Part print with two shaded views. Sizes in mm from the minimum x, y, z corner. A direction names the side the tool comes from. Coordinates: 2 decimals unless noted, no trailing zeros. Write each loop counter-clockwise with the first axis right and the second up, starting at its lowest first coordinate (ties: lowest second). Pieces come first, ordered by that corner, then holes. Notation, with made-up numbers: (10.5, 29.5) - (33.5, 29.5) arc R9 ccw to (33.5, 41.5) - close; hole circle Ø7 at (51.5, 13.5). An arc over 180 degrees is marked (long way). One line per question, with ' | ' between items. Start each with the question number.
1. Probe line 1 (X direction, y = 2.9, z = 3); line 2 (Z direction, x = 69, y = 2.2); line 3 (X direction, y = 2.25, z = 2.5). List the from-to ranges inside material, lowest first.
2. Which spindle directions (+Z, -Z, +X, -X, +Y, -Y) get a long thin tool onto all of the face, cutting with end or side? Do the marked faces 1, 2 and 3. Say none if no direction does.
3. Band-saw the part on C-C, the plane y = 20.75. Write the cut outline in (x, z), then the cut area to 3 significant figures.
4. Flat gauge pins, fed straight in: P1, Ø1.8, axis at x = 4, z = 3, coming from the +Y side; P2, Ø6.5, axis at y = 17, z = 2.5, coming from the -X side; P3, Ø3, axis at x = 3.5, y = 18, coming from the -Z side. Where does each tip first touch, or does it go through?
5. Band-saw the part on A-A, the plane x = 3. Write the cut outline in (y, z), then the cut area to 3 significant figures.
6. Band-saw the part on B-B, the plane z = 47. Write the cut outline in (x, y).
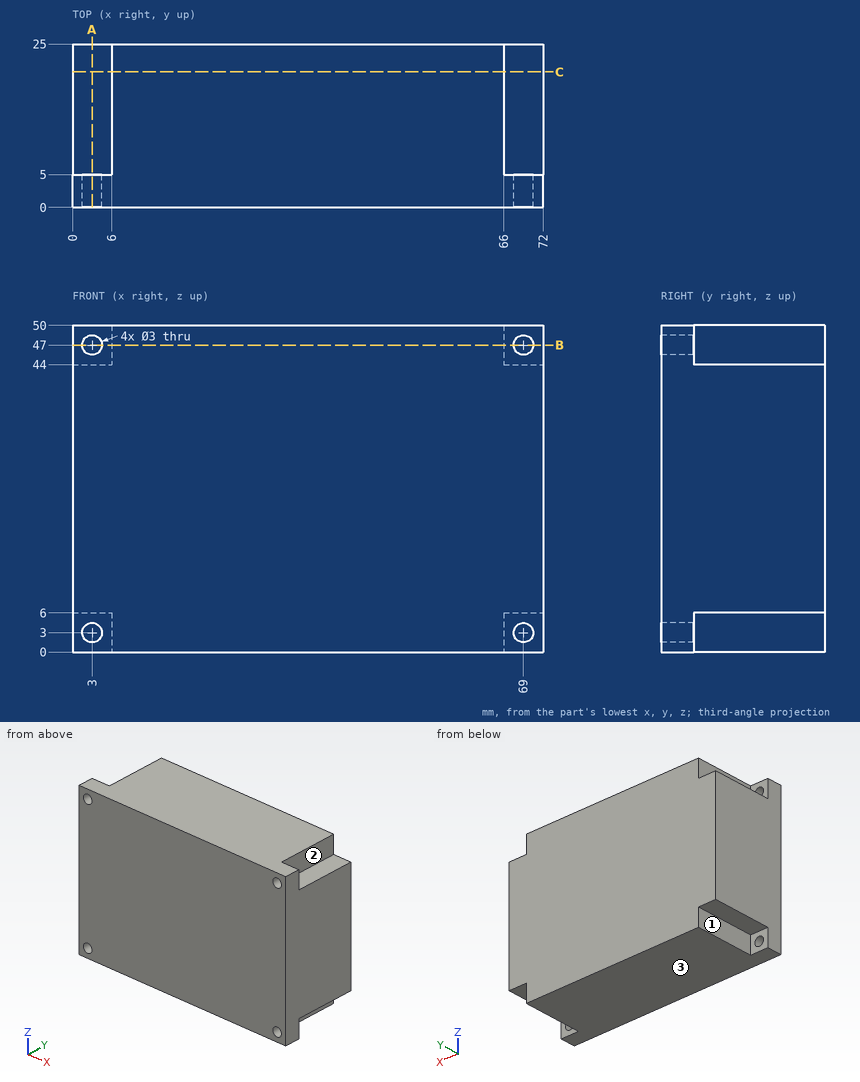
Filled in:
1) line 1: x = 0 to 1.5, 4.5 to 67.5, 70.5 to 72 | line 2: z = 0 to 1.5, 4.5 to 45.5, 48.5 to 50 | line 3: x = 0 to 1.59, 4.41 to 67.59, 70.41 to 72
2) face 1: -Z, -X, +Y | face 2: +Z, +X, +Y | face 3: -Z, +X, -X, +Y, -Y
3) outline: (0, 6) - (6, 6) - (6, 0) - (66, 0) - (66, 6) - (72, 6) - (72, 44) - (66, 44) - (66, 50) - (6, 50) - (6, 44) - (0, 44) - close | area: 3,460 mm²
4) P1: stops at y = 5 | P2: stops at x = 6 | P3: stops at z = 6
5) outline: (0, 0) - (5, 0) - (5, 1.5) - (0, 1.5) - close; (0, 4.5) - (5, 4.5) - (5, 6) - (25, 6) - (25, 44) - (5, 44) - (5, 45.5) - (0, 45.5) - close; (0, 48.5) - (5, 48.5) - (5, 50) - (0, 50) - close | area: 980 mm²
6) outline: (0, 0) - (1.5, 0) - (1.5, 5) - (0, 5) - close; (4.5, 0) - (67.5, 0) - (67.5, 5) - (66, 5) - (66, 25) - (6, 25) - (6, 5) - (4.5, 5) - close; (70.5, 0) - (72, 0) - (72, 5) - (70.5, 5) - close
